Here's how the part is built. I have some questions about the finished solid (model axes, mm). A direction names the side the tool comes from. Give positions to 0.01 mm unless a question says otherwise; leave off trailing zeros. Loops run counter-clockwise (first coordinate to the right, second up) from the corner with the lowest first, then second, coordinate; pieces in that order, holes last.
Q1. Thinking about a two-plate mould opening in X: for faces 4 (the face through (-20, 9, 1)), 5 (the face through (-22, 6, 0)), which applies, pulls with the +X half, pulls with the -X half, needs draft (parallel to the pull), parting line crosses it, or undercut?
Q2. I need wall thicknesses on probe 1 along X at (y, z) = (-0.25, 2.85); probe 2 along Y at (x, z) = (-17.5, 2.55). Which ranges of each line are inside material? Lowest first, please.
Q3. Suppose I cut it at C-C (z = 2.55). Count the separate pieces of the cut face and the enclosed holes in it, and give its area (4 significant figures).
Q4. Suppose I cut it at B-B (x = -8). List the corners of the cut face in (y, z) for me, and give its area (3 significant figures).
Q5. Suppose I cut it at A-A (y = -8). List the corners of the cut face in (x, z) for me.
Q6. For faces 1 (the face through (-20, -5, 1)), 2 (the face through (-10, 9, 1)), 3 (the face through (-33, -10, 1)), which set-ups out of +Z, -Z, +X, -X, +Y, -Y let a thin tool reach every point of the face, with its end or its side?
```python
from build123d import *

# Parameters (mm, degrees)
ESQUISSE1_W        = 5
ESQUISSE1_H        = 3
BOSS_EXTRU_1_DEPTH = 3


with BuildPart() as part:
    # Esquisse1 → Boss.-Extru.1 (new body)
    with BuildSketch(Plane.XY):
        Polygon((-20, -10), (-20, 0), (-15, 0), (-15, -10), (-10, -10), (-10, 0), (-5, 0), (-5, -10), (0, -10), (0, 15.5), (-35, 15.5), (-35, -10), (-30, -10), (-30, 0), (-25, 0), (-25, -10), align=None)
        with Locations((-7.5, 9)):
            Rectangle(ESQUISSE1_W, ESQUISSE1_H, mode=Mode.SUBTRACT)
        with Locations((-17.5, 9)):
            Rectangle(ESQUISSE1_W, ESQUISSE1_H, mode=Mode.SUBTRACT)
        with Locations((-27.5, 9)):
            Rectangle(ESQUISSE1_W, ESQUISSE1_H, mode=Mode.SUBTRACT)
        with Locations((-7.5, 4.5)):
            Rectangle(ESQUISSE1_W, ESQUISSE1_H, mode=Mode.SUBTRACT)
        with Locations((-17.5, 4.5)):
            Rectangle(ESQUISSE1_W, ESQUISSE1_H, mode=Mode.SUBTRACT)
        with Locations((-27.5, 4.5)):
            Rectangle(ESQUISSE1_W, ESQUISSE1_H, mode=Mode.SUBTRACT)
    extrude(amount=BOSS_EXTRU_1_DEPTH)


solid = part.part
```
Solutions:
1. face 4: undercut
1. face 5: needs draft
2. probe 1: x = -35 to -30, -25 to -20, -15 to -10, -5 to 0
2. probe 2: y = 0 to 3, 6 to 7.5, 10.5 to 15.5
3. separate pieces: 1
3. enclosed holes: 6
3. area: 652.5 mm2
4. outline: (0, 0) - (3, 0) - (3, 3) - (0, 3) - close; (6, 0) - (7.5, 0) - (7.5, 3) - (6, 3) - close; (10.5, 0) - (15.5, 0) - (15.5, 3) - (10.5, 3) - close
4. area: 28.5 mm2
5. outline: (-35, 0) - (-30, 0) - (-30, 3) - (-35, 3) - close; (-25, 0) - (-20, 0) - (-20, 3) - (-25, 3) - close; (-15, 0) - (-10, 0) - (-10, 3) - (-15, 3) - close; (-5, 0) - (0, 0) - (0, 3) - (-5, 3) - close
6. face 1: +Z, -Z, -Y
6. face 2: +Z, -Z
6. face 3: +Z, -Z, +X, -X, -Y
